Geometry check sheet. Reference: the model listing, model coordinates, mm. A direction names the side the tool comes from. Round coordinates to 2 decimals unless told otherwise and drop trailing zeros. Order: outer loops, then holes, each group sorted by start corner. A loop starts at its lowest first (then second) coordinate and runs counter-clockwise, first axis right, second up.
(1) Draft check along Y on faces 1 (the face through (18.797, 18.859, -8.337)), 2 (the face through (-12.8, 16.6, 0.8)), 3 (the face through (10, -19, -9)). Enter one of: pulls with the +Y half, pulls with the -Y half, needs draft (parallel to the pull), parting line crosses it, or undercut.
(2) Cross-section at B-B on x = -1.5. Enter the section's corners in (y, z).
(3) Cross-section at D-D on z = -10.75. Enter the section's corners in (x, y), and give its area (3 significant figures).
(4) Gauge pin test, flat ends, axial feed: P1, Ø3, axis at x = -9.5, y = 13.5, coming from the -Z side; P2, Ø0.5, axis at y = -2, z = 1, coming from the -X side; P3, Ø6, axis at y = -5, z = -14, coming from the -X side. Record the tip position at first contact, or that the pin passes through.
(5) Cross-section at A-A on z = 0.5. Enter the section's corners in (x, y).
(6) Cross-section at C-C on y = -8. Enter the section's corners in (x, z).
(7) Thickness scan on L1, parallel to Z at x = 11.5, y = 13; L2, parallel to X at y = 7, z = -3.5; L3, parallel to Y at x = 14, z = -15.75. Record the ranges inside material, lowest first.
(8) Set-up check for faces 4 (the face through (-5, 13, 1)), 5 (the face through (11, -20, -7)), 6 (the face through (10, 19, -9)), 7 (the face through (17.4, 17.43, -9.13)), 8 (the face through (11, 20, -7)): record each of +Z, -Z, +X, -X, +Y, -Y from which the full face is reachable in a straight line by a thin tool's end or side.
from build123d import *

# Parameters (mm, degrees)
F1_DEPTH = 1.6
F2_DEPTH = 18
F3_R     = 4
F4_R     = 2


# Not quite as in the source:
# - a feature names something its author has since deleted; it is built from what else it names


with BuildPart() as f1:
    # F0 (on Top) → F1 (new body)
    with BuildSketch(Plane.XY):
        with BuildLine():
            Line((-9.3, 18.25), (-9.3, 20))
            ThreePointArc((-9.3, 20), (-12.8, 16.5), (-9.3, 13))
            Line((-9.3, 13), (-9.3, 14.75))
            ThreePointArc((-9.3, 14.75), (-11.05, 16.5), (-9.3, 18.25))
        make_face()
        with BuildLine():
            ThreePointArc((-5.8, 16.5), (-6.8251262658, 18.9748737342), (-9.3, 20))
            Line((-9.3, 20), (-9.3, 18.25))
            ThreePointArc((-9.3, 18.25), (-8.0625631329, 17.7374368671), (-7.55, 16.5))
            ThreePointArc((-7.55, 16.5), (-8.0625631329, 15.2625631329), (-9.3, 14.75))
            Line((-9.3, 14.75), (-9.3, 13))
            ThreePointArc((-9.3, 13), (-6.8251262658, 14.0251262658), (-5.8, 16.5))
        make_face()
        with BuildLine():
            Line((0, 13), (0, 20))
            Line((0, 20), (-9.3, 20))
            ThreePointArc((-9.3, 20), (-6.8251262658, 18.9748737342), (-5.8, 16.5))
            ThreePointArc((-5.8, 16.5), (-6.8251262658, 14.0251262658), (-9.3, 13))
            Line((-9.3, 13), (0, 13))
        make_face()
        with BuildLine():
            Line((-9.3, -14.75), (-9.3, -13))
            ThreePointArc((-9.3, -13), (-12.8, -16.5), (-9.3, -20))
            Line((-9.3, -20), (-9.3, -18.25))
            ThreePointArc((-9.3, -18.25), (-11.05, -16.5), (-9.3, -14.75))
        make_face()
        with BuildLine():
            ThreePointArc((-5.8, -16.5), (-6.8251262658, -14.0251262658), (-9.3, -13))
            Line((-9.3, -13), (-9.3, -14.75))
            ThreePointArc((-9.3, -14.75), (-8.0625631329, -15.2625631329), (-7.55, -16.5))
            ThreePointArc((-7.55, -16.5), (-8.0625631329, -17.7374368671), (-9.3, -18.25))
            Line((-9.3, -18.25), (-9.3, -20))
            ThreePointArc((-9.3, -20), (-6.8251262658, -18.9748737342), (-5.8, -16.5))
        make_face()
        with BuildLine():
            Line((0, -20), (0, -13))
            Line((0, -13), (-9.3, -13))
            ThreePointArc((-9.3, -13), (-6.8251262658, -14.0251262658), (-5.8, -16.5))
            ThreePointArc((-5.8, -16.5), (-6.8251262658, -18.9748737342), (-9.3, -20))
            Line((-9.3, -20), (0, -20))
        make_face()
        Polygon((2, 18), (0, 20), (0, 13), (0, -13), (0, -20), (2, -18), align=None)
        Polygon((20, 20), (10, 20), (10, 18), (18, 18), (18, -18), (10, -18), (10, -20), (20, -20), align=None)
        Polygon((10, 18), (2, 18), (2, -18), (10, -18), (18, -18), (18, 18), align=None)
        Polygon((10, 20), (0, 20), (2, 18), (10, 18), align=None)
        Polygon((10, -18), (2, -18), (0, -20), (10, -20), align=None)
    extrude(amount=F1_DEPTH)

    # F0 (on Top) → F2 (join)
    with BuildSketch(Plane.XY):
        Polygon((20, 20), (10, 20), (10, 18), (18, 18), (18, -18), (10, -18), (10, -20), (20, -20), align=None)
    extrude(amount=-F2_DEPTH)

    # F3
    f3_edges = [f1.edges().sort_by_distance(p)[0] for p in [
        (20, -20, -8.2),
        (20, 20, -8.2),
    ]]
    fillet(f3_edges, radius=F3_R)

    # F4
    f4_edges = [f1.edges().sort_by_distance(p)[0] for p in [
        (18, -18, -9),
        (18, 18, -9),
    ]]
    fillet(f4_edges, radius=F4_R)


solid = f1.part
Found:
1. face 1: pulls with the +Y half
1. face 2: undercut
1. face 3: needs draft
2. outline: (-20, 0) - (-13, 0) - (-13, 1.6) - (-20, 1.6) - close; (13, 0) - (20, 0) - (20, 1.6) - (13, 1.6) - close
3. outline: (10, -20) - (16, -20) arc R4 ccw to (20, -16) - (20, 16) arc R4 ccw to (16, 20) - (10, 20) - (10, 18) - (16, 18) arc R2 cw to (18, 16) - (18, -16) arc R2 cw to (16, -18) - (10, -18) - close
3. area: 107 mm2
4. P1: stops at z = 0
4. P2: stops at x = 0
4. P3: stops at x = 18
5. outline: (-9.3, -20) - (16, -20) arc R4 ccw to (20, -16) - (20, 16) arc R4 ccw to (16, 20) - (-9.3, 20) arc R3.5 ccw to (-9.3, 13) - (0, 13) - (0, -13) - (-9.3, -13) arc R3.5 ccw to start; hole circle Ø3.5 at (-9.3, -16.5); hole circle Ø3.5 at (-9.3, 16.5)
6. outline: (0, 0) - (18, 0) - (18, -18) - (20, -18) - (20, 1.6) - (0, 1.6) - close
7. L1: z = 0 to 1.6
7. L2: x = 18 to 20
7. L3: y = -20 to -18, 18 to 20
8. face 4: +Z, -Z, -X
8. face 5: +Z, -Z, +X, -X, -Y
8. face 6: -Z, -X, +Y, -Y
8. face 7: -Z, -X
8. face 8: +Z, -Z, +X, -X, +Y
